from build123d import *

# Parameters (mm, degrees)
SKETCH1_W           = 431.8
SKETCH1_H           = 431.8
BOSS_EXTRUDE1_DEPTH = 6.35
SKETCH2_R           = 79.756
CUT_EXTRUDE1_DEPTH  = 6.35
CUT_EXTRUDE2_DEPTH  = 6.35
FILLET1_R           = 12.7
SKETCH4_R           = 3.175
CUT_EXTRUDE3_DEPTH  = 6.35


with BuildPart() as part:
    # Sketch1 → Boss-Extrude1 (new body)
    with BuildSketch(Plane.XY):
        Rectangle(SKETCH1_W, SKETCH1_H)
    extrude(amount=BOSS_EXTRUDE1_DEPTH)

    # Sketch2 → Cut-Extrude1 (cut)
    with BuildSketch(Plane.XY.offset(6.35)):
        Circle(SKETCH2_R)
    extrude(amount=-CUT_EXTRUDE1_DEPTH, mode=Mode.SUBTRACT)

    # Sketch3 → Cut-Extrude2 (cut)
    with BuildSketch(Plane.XY.offset(6.35)):
        Polygon((-170.804471423, 175.474204606), (-175.474204606, 170.804471423), (-55.532184739, 50.862451556), (-50.862451556, 55.532184739), align=None)
        Polygon((175.474204606, 170.804471423), (170.804471423, 175.474204606), (50.862451556, 55.532184739), (55.532184739, 50.862451556), align=None)
        Polygon((170.804471423, -175.474204606), (175.474204606, -170.804471423), (55.532184739, -50.862451556), (50.862451556, -55.532184739), align=None)
        Polygon((-175.474204606, -170.804471423), (-170.804471423, -175.474204606), (-50.862451556, -55.532184739), (-55.532184739, -50.862451556), align=None)
    extrude(amount=-CUT_EXTRUDE2_DEPTH, mode=Mode.SUBTRACT)

    # Fillet1
    fillet1_edges = [part.edges().sort_by_distance(p)[0] for p in [
        (-54.012787894, 58.682521077, 3.175),
        (-58.682521077, 54.012787894, 3.175),
        (58.682521077, 54.012787894, 3.175),
        (54.012787894, 58.682521077, 3.175),
        (54.012787894, -58.682521077, 3.175),
        (58.682521077, -54.012787894, 3.175),
        (-58.682521077, -54.012787894, 3.175),
        (-54.012787894, -58.682521077, 3.175),
    ]]
    fillet(fillet1_edges, radius=FILLET1_R)

    # Sketch4 → Cut-Extrude3 (cut)
    with BuildSketch(Plane.XY.offset(6.35)):
        with Locations((0, 139.7)):
            Circle(SKETCH4_R)
        with Locations((139.7, 0)):
            Circle(SKETCH4_R)
        with Locations((0, -139.7)):
            Circle(SKETCH4_R)
        with Locations((-139.7, 0)):
            Circle(SKETCH4_R)
    extrude(amount=-CUT_EXTRUDE3_DEPTH, mode=Mode.SUBTRACT)


solid = part.part
Work out the finished part from the listing and answer in its coordinate system (mm). A direction names the side the tool comes from. Give positions to 0.01 mm unless a question says otherwise; leave off trailing zeros. Loops run counter-clockwise (first coordinate to the right, second up) from the corner with the lowest first, then second, coordinate; pieces in that order, holes last. Notation, with made-up numbers: (-17, 9.25) - (19, 9.25) arc R11 cw to (19, 21.25) - close; hole circle Ø4 at (58, -19). An arc over 180 degrees is marked (long way). Answer in a Markdown table with one row per item. Add a question column.
Q1. Determine the mould class of faces 1 (the flat face through (120.34, 115.67, 3.22)), 2 (the flat face through (93, 3, 0)) for opening direction Y: released by +Y, released by -Y, zero draft, split by the parting line, or undercut.
Q2. Consider line 1 along Y through (x, z) = (0, 5) (3 decimals); line 2 along X through (y, z) = (-139.7, 3.5) (3 decimals); line 3 along X through (y, z) = (107.5, 4). Determine where each line is inside the solid, lowest interval first.
Q3. The part is cut by section C-C (z = 4.75). State how many separate pieces and enclosed holes the cut face has, and give its area (3 significant figures).
Q4. The part is cut by section A-A (y = -8.5). Determine the outline of the cut face in (x, z), and give its area (3 significant figures).
Q5. A tool of negligible diameter and unlimited length cuts with its end or side. For faces 3 (the cylindrical face through (0.683, 79.753, 3.219)), 4 (the flat face through (93, 3, 6.35)), from which of +Z, -Z, +X, -X, +Y, -Y can it reach the whole face along a straight path? Write none if from no direction.
Q6. This flat-tipped pin is pushed along its axis until it touches: P1, Ø5, axis at x = 139.7, y = 0, coming from the +Z side. Where does it stop, or does it pass through?
Q7. The part is cut by section D-D (y = 104). Determine the outline of the cut face in (x, z).
Q8. The part is cut by section B-B (x = -85). Determine the outline of the cut face in (y, z).
Solution:
| question | item | result |
|---|---|---|
| 1 | face 1 | undercut |
| 1 | face 2 | zero draft |
| 2 | line 1 | y = -215.9 to -142.875, -136.525 to -79.756, 79.756 to 136.525, 142.875 to 215.9 |
| 2 | line 2 | x = -215.9 to -144.37, -135.03 to -3.175, 3.175 to 135.03, 144.37 to 215.9 |
| 2 | line 3 | x = -215.9 to -112.17, -102.83 to 102.83, 112.17 to 215.9 |
| 3 | separate pieces | 1 |
| 3 | enclosed holes | 5 |
| 3 | area | 162,000 mm² |
| 4 | outline | (-215.9, 0) - (-79.3, 0) - (-79.3, 6.35) - (-215.9, 6.35) - close; (79.3, 0) - (215.9, 0) - (215.9, 6.35) - (79.3, 6.35) - close |
| 4 | area | 1,730 mm² |
| 5 | face 3 | +Z, -Z |
| 5 | face 4 | +Z, +X, -X, +Y, -Y |
| 6 | P1 | passes through |
| 7 | outline | (-215.9, 0) - (-108.67, 0) - (-108.67, 6.35) - (-215.9, 6.35) - close; (-99.33, 0) - (99.33, 0) - (99.33, 6.35) - (-99.33, 6.35) - close; (108.67, 0) - (215.9, 0) - (215.9, 6.35) - (108.67, 6.35) - close |
| 8 | outline | (-215.9, 0) - (-89.67, 0) - (-89.67, 6.35) - (-215.9, 6.35) - close; (-80.33, 0) - (80.33, 0) - (80.33, 6.35) - (-80.33, 6.35) - close; (89.67, 0) - (215.9, 0) - (215.9, 6.35) - (89.67, 6.35) - close |
